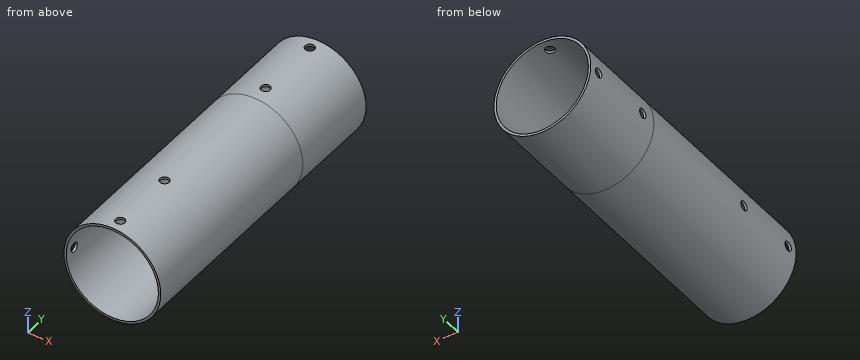
```python
from build123d import *

# Parameters (mm, degrees)
F2_R      = 20.8464397385
F2_R_2    = 19.8464397385
F3_DEPTH  = 25
F4_R      = 20.8464397385
F4_R_2    = 19.8464397385
F5_DEPTH  = 40
F8_R      = 20.8464397385
F8_R_2    = 19.8464397385
F9_DEPTH  = 40
F6_R      = 2
F10_DEPTH = 20.8474397385
F7_R      = 2
F11_DEPTH = 20.8474398385
F12_R     = 2
F13_DEPTH = 20.8474398715
F14_R     = 2
F15_DEPTH = 20.8474398385


with BuildPart() as f3:
    # F2 (on Front) → F3 (new body, symmetric)
    with BuildSketch(Plane.XZ):
        Circle(F2_R)
        Circle(F2_R_2, mode=Mode.SUBTRACT)
    extrude(amount=F3_DEPTH, both=True)

    # F4 (on face) → F5 (join)
    with BuildSketch(Plane.XZ.offset(25)):
        Circle(F4_R)
        Circle(F4_R_2, mode=Mode.SUBTRACT)
    extrude(amount=F5_DEPTH)

    # F8 (on face) → F9 (join)
    with BuildSketch(Plane(origin=(0, 25, 0), x_dir=(-1, 0, 0), z_dir=(0, 1, 0))):
        Circle(F8_R)
        Circle(F8_R_2, mode=Mode.SUBTRACT)
    extrude(amount=F9_DEPTH)

    # F6 (on Top) → F10 (cut, through all)
    with BuildSketch(Plane.XY):
        with Locations((0, -32)):
            Circle(F6_R)
        with Locations((0, -60)):
            Circle(F6_R)
    extrude(amount=F10_DEPTH, mode=Mode.SUBTRACT)

    # F7 (on Right) → F11 (cut, through all)
    with BuildSketch(Plane.YZ):
        with Locations((-60, 0)):
            Circle(F7_R)
        with Locations((-32, 0)):
            Circle(F7_R)
    extrude(amount=-F11_DEPTH, mode=Mode.SUBTRACT)

    # F12 (on Top) → F13 (cut, through all)
    with BuildSketch(Plane.XY):
        with Locations((0, 60)):
            Circle(F12_R)
        with Locations((0, 32)):
            Circle(F12_R)
    extrude(amount=F13_DEPTH, mode=Mode.SUBTRACT)

    # F14 (on Right) → F15 (cut, through all)
    with BuildSketch(Plane.YZ):
        with Locations((60, 0)):
            Circle(F14_R)
        with Locations((32, 0)):
            Circle(F14_R)
    extrude(amount=-F15_DEPTH, mode=Mode.SUBTRACT)


solid = f3.part
```
Verification items for the finished model (mm, model axes). Coordinates: 2 decimals unless noted, no trailing zeros. Order: outer loops, then holes, each group sorted by start corner. A loop starts at its lowest first (then second) coordinate and runs counter-clockwise, first axis right, second up. Notation, with made-up numbers: (33.5, 65.5) - (77.5, 65.5) arc R14 cw to (77.5, 90.5) - close; hole circle Ø5 at (-31, 52). An arc over 180 degrees is marked (long way). Return JSON: item names as keys, results as strings.
(1) Section check A-A, the plane x = 0. Record the cut outline in (y, z), and give its area (3 significant figures).
Filled sheet:
{"outline": "(-65, -20.85) - (65, -20.85) - (65, -19.85) - (-65, -19.85) - close; (-65, 19.85) - (-62, 19.85) - (-62, 20.85) - (-65, 20.85) - close; (-58, 19.85) - (-34, 19.85) - (-34, 20.85) - (-58, 20.85) - close; (-30, 19.85) - (30, 19.85) - (30, 20.85) - (-30, 20.85) - close; (34, 19.85) - (58, 19.85) - (58, 20.85) - (34, 20.85) - close; (62, 19.85) - (65, 19.85) - (65, 20.85) - (62, 20.85) - close", "area": "244 mm^2"}
(2) Thickness scan on line 1 along Z through (x, y) = (0, -16); line 2 along Z through (x, y) = (-3.5, 25.5). Record the ranges inside material, lowest first.
Filled sheet:
{"line 1": "z = -20.85 to -19.85, 19.85 to 20.85", "line 2": "z = -20.55 to -19.54, 19.54 to 20.55"}
(3) Go/stop test with flat-tipped pins: pin 1 (6 mm diameter, centred on x = -10.5, y = -21.5, fed in from -Z); pin 2 (2 mm diameter, centred on x = 3, y = -8, fed in from -Z); pin 3 (2.5 mm diameter, centred on y = 32, z = 0, fed in from -X). Record where each tip stops, or that it passes through.
Filled sheet:
{"pin 1": "stops at z = -19.45", "pin 2": "stops at z = -20.75", "pin 3": "stops at x = 19.81"}
(4) Section check D-D, the plane x = 10. Record the cut outline in (y, z).
Filled sheet:
{"outline": "(-65, -18.29) - (65, -18.29) - (65, -17.14) - (-65, -17.14) - close; (-65, 17.14) - (65, 17.14) - (65, 18.29) - (-65, 18.29) - close"}
(5) Section check C-C, the plane y = 32. Record the cut outline in (x, z), and give its area (3 significant figures).
Filled sheet:
{"outline": "(-20.75, -2) arc R20.85 ccw (long way) to (2, 20.75) - (2, 19.75) arc R19.85 cw (long way) to (-19.75, -2) - close; (-20.75, 2) - (-19.75, 2) arc R19.85 cw to (-2, 19.75) - (-2, 20.75) arc R20.85 ccw to start", "area": "120 mm^2"}
(6) Section check B-B, the plane z = 0. Record the cut outline in (x, y), and give its area (3 significant figures).
Filled sheet:
{"outline": "(-20.85, -65) - (-19.85, -65) - (-19.85, -62) - (-20.85, -62) - close; (-20.85, -58) - (-19.85, -58) - (-19.85, -34) - (-20.85, -34) - close; (-20.85, -30) - (-19.85, -30) - (-19.85, 30) - (-20.85, 30) - close; (-20.85, 34) - (-19.85, 34) - (-19.85, 58) - (-20.85, 58) - close; (-20.85, 62) - (-19.85, 62) - (-19.85, 65) - (-20.85, 65) - close; (19.85, -65) - (20.85, -65) - (20.85, 65) - (19.85, 65) - close", "area": "244 mm^2"}
